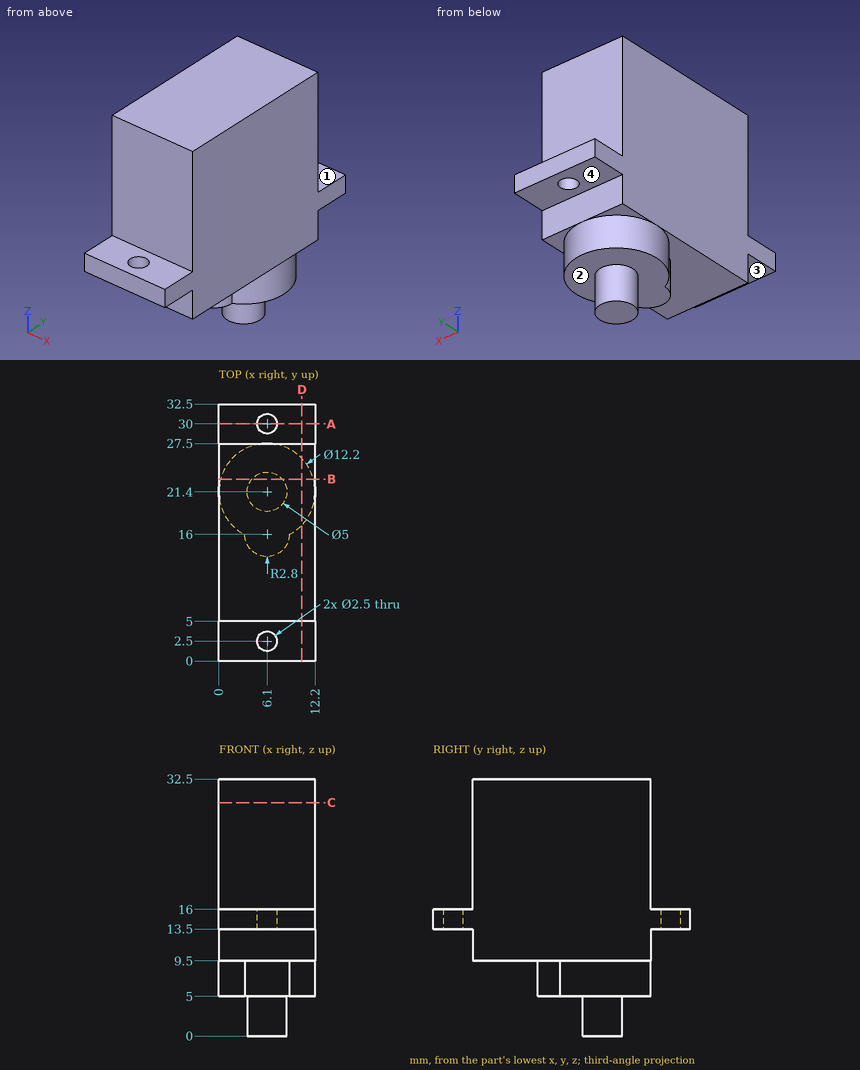
Input: dimensioned drawing with shaded views. Units: mm. Origin: part minimum x, y, z. A direction names the side the tool comes from. Give positions to 0.01 mm unless a question says otherwise; leave off trailing zeros. Write each loop counter-clockwise with the first axis right and the second up, starting at its lowest first coordinate (ties: lowest second). Pieces come first, ordered by that corner, then holes.
1. Line query: probe 1 along Y at (x, z) = (6.1, 15.35); probe 2 along Z at (x, y) = (1.75, 21.5); probe 3 along Y at (x, z) = (8.5, 25). Output: solid intervals per line, ascending.
2. Pin query (flat end, axial travel): P1, Ø1, axis at x = 9.5, y = 10, coming from the -Z side; P2, Ø5, axis at x = 10, y = 25.5, coming from the -Z side; P3, Ø1.5, axis at x = 10, y = 3.5, coming from the +Z side; P4, Ø2, axis at x = 6.1, y = 30, coming from the -Z side. Return the tip coordinate at first contact, or that it passes through.
3. Section query A-A, the plane y = 30. Return loops of the section in (x, z).
4. Reachability of the marked faces 1, 2, 3 and 4 from +Z, -Z, +X, -X, +Y, -Y: full face, straight path, thin tool, end or side. Return the list, or none.
5. Section query C-C, the plane z = 29.5. Return loops of the section in (x, y).
6. Section query B-B, the plane y = 23. Return loops of the section in (x, z).
7. Section query D-D, the plane x = 10.5. Return loops of the section in (y, z).
Computed:
1. probe 1: y = 0 to 1.25, 3.75 to 28.75, 31.25 to 32.5
1. probe 2: z = 5 to 32.5
1. probe 3: y = 5 to 27.5
2. P1: stops at z = 9.5
2. P2: stops at z = 5
2. P3: stops at z = 16
2. P4: passes through
3. outline: (0, 13.5) - (4.85, 13.5) - (4.85, 16) - (0, 16) - close; (7.35, 13.5) - (12.2, 13.5) - (12.2, 16) - (7.35, 16) - close
4. face 1: +Z, +X, -X, +Y
4. face 2: -Z
4. face 3: -Z, +X, -X, -Y
4. face 4: -Z, +X, -X, +Y
5. outline: (0, 5) - (12.2, 5) - (12.2, 27.5) - (0, 27.5) - close
6. outline: (0, 9.5) - (0.21, 9.5) - (0.21, 5) - (4.18, 5) - (4.18, 0) - (8.02, 0) - (8.02, 5) - (11.99, 5) - (11.99, 9.5) - (12.2, 9.5) - (12.2, 32.5) - (0, 32.5) - close
7. outline: (0, 13.5) - (5, 13.5) - (5, 9.5) - (17.18, 9.5) - (17.18, 5) - (25.62, 5) - (25.62, 9.5) - (27.5, 9.5) - (27.5, 13.5) - (32.5, 13.5) - (32.5, 16) - (27.5, 16) - (27.5, 32.5) - (5, 32.5) - (5, 16) - (0, 16) - close
